```python
from build123d import *

# Parameters (mm, degrees)
ESBO_O1_W                                   = 75
ESBO_O1_H                                   = 30
RESSALTO_EXTRUS_O1_DEPTH                    = 10.7
ESBO_O2_R                                   = 6
CORTE_EXTRUS_O1_DEPTH                       = 11.7
ESBO_O7_R                                   = 11
CORTE_EXTRUS_O6_DEPTH                       = 11.7
FURO_ROSCADO_PARA_CONDU_TE_DE_1_4_281_D     = 6.6294
FURO_ROSCADO_PARA_CONDU_TE_DE_1_4_281_DEPTH = 15
FURO_ROSCADO_PARA_CONDU_TE_DE_1_4_281_TIP   = 1.991672694
FURO_ROSCADO_PARA_CONDU_TE_DE_1_4_282_D     = 6.6294
FURO_ROSCADO_PARA_CONDU_TE_DE_1_4_282_DEPTH = 15
FURO_ROSCADO_PARA_CONDU_TE_DE_1_4_282_TIP   = 1.991672694
FURO_ROSCADO_PARA_CONDU_TE_DE_1_4_283_D     = 6.6294
FURO_ROSCADO_PARA_CONDU_TE_DE_1_4_283_DEPTH = 15
FURO_ROSCADO_PARA_CONDU_TE_DE_1_4_283_TIP   = 1.991672694
FURO_ROSCADO_PARA_CONDU_TE_DE_1_4_284_D     = 6.6294
FURO_ROSCADO_PARA_CONDU_TE_DE_1_4_284_DEPTH = 12
FURO_ROSCADO_PARA_CONDU_TE_DE_1_4_284_TIP   = 1.991672694


with BuildPart() as part:
    # Esboço1 → Ressalto-extrusão1 (new body)
    with BuildSketch(Plane.XY):
        Rectangle(ESBO_O1_W, ESBO_O1_H)
    extrude(amount=RESSALTO_EXTRUS_O1_DEPTH)

    # Esboço2 → Corte-extrusão1 (cut, through all)
    with BuildSketch(Plane.XY.offset(10.7)):
        with Locations((-24, 0)):
            Circle(ESBO_O2_R)
        with Locations((24, 0)):
            Circle(ESBO_O2_R)
    extrude(amount=-CORTE_EXTRUS_O1_DEPTH, mode=Mode.SUBTRACT)

    # Esboço7 → Corte-extrusão6 (cut, through all)
    with BuildSketch(Plane.XY.offset(10.7)):
        Circle(ESBO_O7_R)
    extrude(amount=-CORTE_EXTRUS_O6_DEPTH, mode=Mode.SUBTRACT)

    # Furo roscado para conduíte de 1/4-281
    with Locations(Plane(origin=(0, 15, 0), x_dir=(1, 0, 0), z_dir=(0, 1, 0))):
        with Locations((-24, -5.35), (24, -5.35)):
            Hole(FURO_ROSCADO_PARA_CONDU_TE_DE_1_4_281_D / 2, depth=FURO_ROSCADO_PARA_CONDU_TE_DE_1_4_281_DEPTH)
            with Locations((0, 0, -(FURO_ROSCADO_PARA_CONDU_TE_DE_1_4_281_DEPTH + FURO_ROSCADO_PARA_CONDU_TE_DE_1_4_281_TIP / 2))):  # 118° drill point
                Cone(0, FURO_ROSCADO_PARA_CONDU_TE_DE_1_4_281_D / 2, FURO_ROSCADO_PARA_CONDU_TE_DE_1_4_281_TIP, mode=Mode.SUBTRACT)

    # Furo roscado para conduíte de 1/4-282
    with Locations(Plane.ZY.offset(37.5)):
        with Locations((5.35, 0)):
            Hole(FURO_ROSCADO_PARA_CONDU_TE_DE_1_4_282_D / 2, depth=FURO_ROSCADO_PARA_CONDU_TE_DE_1_4_282_DEPTH)
            with Locations((0, 0, -(FURO_ROSCADO_PARA_CONDU_TE_DE_1_4_282_DEPTH + FURO_ROSCADO_PARA_CONDU_TE_DE_1_4_282_TIP / 2))):  # 118° drill point
                Cone(0, FURO_ROSCADO_PARA_CONDU_TE_DE_1_4_282_D / 2, FURO_ROSCADO_PARA_CONDU_TE_DE_1_4_282_TIP, mode=Mode.SUBTRACT)

    # Furo roscado para conduíte de 1/4-283
    with Locations(Plane(origin=(37.5, 0, 0), x_dir=(0, 0, -1), z_dir=(1, 0, 0))):
        with Locations((-5.35, 0)):
            Hole(FURO_ROSCADO_PARA_CONDU_TE_DE_1_4_283_D / 2, depth=FURO_ROSCADO_PARA_CONDU_TE_DE_1_4_283_DEPTH)
            with Locations((0, 0, -(FURO_ROSCADO_PARA_CONDU_TE_DE_1_4_283_DEPTH + FURO_ROSCADO_PARA_CONDU_TE_DE_1_4_283_TIP / 2))):  # 118° drill point
                Cone(0, FURO_ROSCADO_PARA_CONDU_TE_DE_1_4_283_D / 2, FURO_ROSCADO_PARA_CONDU_TE_DE_1_4_283_TIP, mode=Mode.SUBTRACT)

    # Furo roscado para conduíte de 1/4-284
    with Locations(Plane(origin=(0, -15, 0), x_dir=(-1, 0, 0), z_dir=(0, -1, 0))):
        with Locations((15, -5.35), (-15, -5.35)):
            Hole(FURO_ROSCADO_PARA_CONDU_TE_DE_1_4_284_D / 2, depth=FURO_ROSCADO_PARA_CONDU_TE_DE_1_4_284_DEPTH)
            with Locations((0, 0, -(FURO_ROSCADO_PARA_CONDU_TE_DE_1_4_284_DEPTH + FURO_ROSCADO_PARA_CONDU_TE_DE_1_4_284_TIP / 2))):  # 118° drill point
                Cone(0, FURO_ROSCADO_PARA_CONDU_TE_DE_1_4_284_D / 2, FURO_ROSCADO_PARA_CONDU_TE_DE_1_4_284_TIP, mode=Mode.SUBTRACT)


solid = part.part
```
For this review, take the finished solid that the model builds, in its own axes (mm). A direction names the side the tool comes from. Coordinates: 2 decimals unless noted, no trailing zeros. Write each loop counter-clockwise with the first axis right and the second up, starting at its lowest first coordinate (ties: lowest second). Pieces come first, ordered by that corner, then holes. Notation, with made-up numbers: (-30.75, -4) - (22.25, -4) arc R30 cw to (22.25, 23) - close; hole circle Ø11 at (-5.75, 51). An arc over 180 degrees is marked (long way). Put each result on its own line as item: value.
1. Add section C-C, the plane x = 24. Give the boundary of the cut face in (y, z), then the cut area to 3 significant figures.
Values found:
outline: (-15, 0) - (-6, 0) - (-6, 10.7) - (-15, 10.7) - close; (6, 0) - (15, 0) - (15, 2.04) - (6, 2.04) - close; (6, 8.66) - (15, 8.66) - (15, 10.7) - (6, 10.7) - close
area: 133 mm²
2. Add section B-B, the plane y = 7. Give the boundary of the cut face in (x, z), then the cut area to 3 significant figures.
Values found:
outline: (-37.5, 0) - (-8.49, 0) - (-8.49, 10.7) - (-37.5, 10.7) - close; (8.49, 0) - (37.5, 0) - (37.5, 10.7) - (8.49, 10.7) - close; hole circle Ø6.63 at (-24, 5.35); hole circle Ø6.63 at (24, 5.35)
area: 552 mm²
3. Machinability: for faces 1 (the cylindrical face through (19.24, -3.65, 5.42)), 2 (the flat face through (-1, -15, 5)), 3 (the cylindrical face through (12.557, -8.916, 3.11)), 4 (the cylindrical face through (27.31, 9.93, 5.2)), 5 (the cylindrical face through (33.2, -1.3, 8.4)), which of the approach directions +Z, -Z, +X, -X, +Y, -Y give a long, thin tool a straight path to every point of the face, cutting with its end or side? Answer none if there is none.
Values found:
face 1: +Z, -Z
face 2: +Z, -Z, +X, -X, -Y
face 3: -Y
face 4: +Y
face 5: +X
4. Add section D-D, the plane y = 0. Give the boundary of the cut face in (x, z).
Values found:
outline: (-37.5, 0) - (-30, 0) - (-30, 2.04) - (-37.5, 2.04) - close; (-37.5, 8.66) - (-30, 8.66) - (-30, 10.7) - (-37.5, 10.7) - close; (-18, 0) - (-11, 0) - (-11, 10.7) - (-18, 10.7) - close; (11, 0) - (18, 0) - (18, 10.7) - (11, 10.7) - close; (30, 0) - (37.5, 0) - (37.5, 2.04) - (30, 2.04) - close; (30, 8.66) - (37.5, 8.66) - (37.5, 10.7) - (30, 10.7) - close
5. Wall thickness on probe 1 along Y at (x, z) = (32.25, 5.35); probe 2 along Z at (x, y) = (-15, -12.25); probe 3 along X at (y, z) = (-4, 2.5): over which ranges is each line inside the solid? List them lowest first.
Values found:
probe 1: -15 to -3.31, 3.31 to 15
probe 2: 0 to 2.04, 8.66 to 10.7
probe 3: -37.5 to -28.47, -19.53 to -16.69, -13.31 to -10.25, 10.25 to 13.31, 16.69 to 19.53, 28.47 to 37.5
6. Mouldability with a two-part tool opening along Y and no side actions: class faces 6 (the conical face through (-15.309, -1.354, 4.865)), 7 (the cylindrical face through (-33.19, 1, 2.19)), 8 (the cylindrical face through (-20.69, 9.93, 5.2)) as released by +Y, released by -Y, zero draft, split by the parting line, or undercut.
Values found:
face 6: released by -Y
face 7: undercut
face 8: zero draft
7. For pin 1 (5.5 mm diameter, centred on y = 0, z = 5.35, fed in from -X); pin 2 (6 mm diameter, centred on y = 0, z = 5.35, fed in from -X), all flat-tipped, find the tip position at first contact; note any pin that passes through.
Values found:
pin 1: x = -18.67
pin 2: x = -18.8
8. Add section A-A, the plane x = 0. Give the boundary of the cut face in (y, z), then the cut area to 3 significant figures.
Values found:
outline: (-15, 0) - (-11, 0) - (-11, 10.7) - (-15, 10.7) - close; (11, 0) - (15, 0) - (15, 10.7) - (11, 10.7) - close
area: 85.6 mm²
